from build123d import *
from OCP.BRepFilletAPI import BRepFilletAPI_MakeChamfer

# Parameters (mm, degrees)
BASE_W               = 85
BASE_H               = 100
BOSS_EXTRUDE2_DEPTH  = 2
SKETCH3_W            = 9
SKETCH3_H            = 1.5
SKETCH3_W_2          = 43
SKETCH3_H_2          = 2.5
BOSS_EXTRUDE4_DEPTH  = 11
SKETCH13_W           = 15
SKETCH13_H           = 61.230763763
SKETCH13_R           = 1
CUT_EXTRUDE2_DEPTH   = 67.537583365
SKETCH14_W           = 2.595547293
SKETCH14_H           = 6.5
SKETCH14_W_2         = 6.5
SKETCH14_H_2         = 2
BOSS_EXTRUDE5_DEPTH  = 25
SKETCH16_W           = 3.995410841
SKETCH16_H           = 2.5
BOSS_EXTRUDE6_DEPTH  = 29
SKETCH18_W           = 4
SKETCH18_H           = 6.5
BOSS_EXTRUDE7_DEPTH  = 40
CHAMFER1_SIZE        = 8.502262467
CHAMFER1_SIZE_2      = 40
SKETCH19_W           = 10.5
SKETCH19_H           = 63.5
CUT_EXTRUDE3_DEPTH   = 77.852130745
BOSS_EXTRUDE8_DEPTH  = 5
FILLET1_R            = 10
SKETCH21_W           = 2
SKETCH21_H           = 2
BOSS_EXTRUDE9_DEPTH  = 3.4
SKETCH22_W           = 64
SKETCH22_H           = 2
BOSS_EXTRUDE10_DEPTH = 35
SKETCH23_R           = 1.5
SKETCH23_W           = 30
SKETCH23_H           = 27.486629776
CUT_EXTRUDE4_DEPTH   = 104.107953137
SKETCH24_W           = 1
SKETCH24_H           = 32.46
SKETCH24_W_2         = 10
SKETCH24_H_2         = 1
BOSS_EXTRUDE11_DEPTH = 5
SKETCH26_W           = 2
SKETCH26_H           = 2
BOSS_EXTRUDE13_DEPTH = 3.4


with BuildPart() as part:
    # base → Boss-Extrude2 (new body)
    with BuildSketch(Plane(origin=(0, 0, 0), x_dir=(1, 0, 0), z_dir=(0, 1, 0))):
        Rectangle(BASE_W, BASE_H)
    extrude(amount=BOSS_EXTRUDE2_DEPTH)

    # Sketch3 → Boss-Extrude4 (add)
    with BuildSketch(Plane(origin=(0, 2, 0), x_dir=(1, 0, 0), z_dir=(0, 1, 0))):
        with Locations((38, 41.25)):
            Rectangle(SKETCH3_W, SKETCH3_H)
        with Locations((38, 27.75)):
            Rectangle(SKETCH3_W, SKETCH3_H)
        with Locations((-38, 41.25)):
            Rectangle(SKETCH3_W, SKETCH3_H)
        with Locations((-38, 27.75)):
            Rectangle(SKETCH3_W, SKETCH3_H)
        with Locations((0, 41.75)):
            Rectangle(SKETCH3_W_2, SKETCH3_H_2)
    extrude(amount=BOSS_EXTRUDE4_DEPTH)

    # Sketch13 → Cut-Extrude2 (cut, through all)
    with BuildSketch(Plane(origin=(0, 2, 0), x_dir=(1, 0, 0), z_dir=(0, 1, 0))):
        with BuildLine():
            ThreePointArc((-16.872793903, 34.5), (-13.024991104, 30.652197201), (-9.177188305, 34.5))
            Line((-9.177188305, 34.5), (-16.872793903, 34.5))
        make_face()
        with BuildLine():
            Line((-16.872793903, 34.5), (-9.177188305, 34.5))
            ThreePointArc((-9.177188305, 34.5), (-13.024991104, 38.347802799), (-16.872793903, 34.5))
        make_face()
        with BuildLine():
            ThreePointArc((9.177188305, 34.5), (13.024991104, 30.652197201), (16.872793903, 34.5))
            Line((16.872793903, 34.5), (9.177188305, 34.5))
        make_face()
        with BuildLine():
            Line((9.177188305, 34.5), (16.872793903, 34.5))
            ThreePointArc((16.872793903, 34.5), (13.024991104, 38.347802799), (9.177188305, 34.5))
        make_face()
        with Locations((-7.5, -19.384618119)):
            Rectangle(SKETCH13_W, SKETCH13_H)
        with Locations((7.5, -19.384618119)):
            Rectangle(SKETCH13_W, SKETCH13_H)
        with Locations(Location((28.5, 45, 0), (0, 0, 270))):
            Circle(SKETCH13_R)
        with Locations(Location((28.5, 24, 0), (0, 0, 90))):
            Circle(SKETCH13_R)
        with Locations(Location((-28.5, 24, 0), (0, 0, 270))):
            Circle(SKETCH13_R)
        with Locations(Location((-28.5, 45, 0), (0, 0, 90))):
            Circle(SKETCH13_R)
    extrude(amount=-CUT_EXTRUDE2_DEPTH, mode=Mode.SUBTRACT)

    # Sketch14 → Boss-Extrude5 (add)
    with BuildSketch(Plane(origin=(0, 2, 0), x_dir=(1, 0, 0), z_dir=(0, 1, 0))):
        with Locations((-36.123593927, 23.75)):
            Rectangle(SKETCH14_W, SKETCH14_H)
        with Locations((-34.171367573, 19.5)):
            Rectangle(SKETCH14_W_2, SKETCH14_H_2)
        with Locations((36.123593927, 23.75)):
            Rectangle(SKETCH14_W, SKETCH14_H)
        Polygon((37.421367573, 20.5), (34.82582028, 20.5), (30.921367573, 20.5), (30.921367573, 18.5), (37.421367573, 18.5), align=None)
    extrude(amount=BOSS_EXTRUDE5_DEPTH)

    # Sketch16 → Boss-Extrude6 (add)
    with BuildSketch(Plane(origin=(0, 13, 0), x_dir=(1, 0, 0), z_dir=(0, 1, 0))):
        with Locations((-19.50229458, 41.75)):
            Rectangle(SKETCH16_W, SKETCH16_H)
        with Locations((19.50229458, 41.75)):
            Rectangle(SKETCH16_W, SKETCH16_H)
    extrude(amount=BOSS_EXTRUDE6_DEPTH)

    # Sketch18 → Boss-Extrude7 (add)
    with BuildSketch(Plane(origin=(0, 2, 0), x_dir=(1, 0, 0), z_dir=(0, 1, 0))):
        with Locations((-19.5, 46.25)):
            Rectangle(SKETCH18_W, SKETCH18_H)
        with Locations((19.5, 46.25)):
            Rectangle(SKETCH18_W, SKETCH18_H)
    extrude(amount=BOSS_EXTRUDE7_DEPTH)

    # Chamfer1
    chamfer1_edges_1 = [part.edges().sort_by_distance(p)[0] for p in [
        (-19.5, 42, -49.5),
    ]]
    chamfer1_side_1 = [part.faces().sort_by_distance(p)[0] for p in [
        (-19.5, 42, -49.329954751),
    ]]
    chamfer1_edges_2 = [part.edges().sort_by_distance(p)[0] for p in [
        (19.5, 42, -49.5),
    ]]
    chamfer1_side_2 = [part.faces().sort_by_distance(p)[0] for p in [
        (19.5, 42, -49.329954751),
    ]]
    chamfer1 = BRepFilletAPI_MakeChamfer(part.part.solid().wrapped)
    for e in chamfer1_edges_1:
        chamfer1.Add(CHAMFER1_SIZE - 0.0001, CHAMFER1_SIZE_2 - 0.0001, e.wrapped, chamfer1_side_1[0].wrapped)
    for e in chamfer1_edges_2:
        chamfer1.Add(CHAMFER1_SIZE - 0.0001, CHAMFER1_SIZE_2 - 0.0001, e.wrapped, chamfer1_side_2[0].wrapped)
    add(Compound.cast(chamfer1.Shape()), mode=Mode.REPLACE)  # a hair under: the kernel refuses the full size

    # Sketch19 → Cut-Extrude3 (cut, through all)
    with BuildSketch(Plane(origin=(0, 2, 0), x_dir=(1, 0, 0), z_dir=(0, 1, 0))):
        with Locations((-37.25, -18.25)):
            Rectangle(SKETCH19_W, SKETCH19_H)
        with Locations((37.25, -18.25)):
            Rectangle(SKETCH19_W, SKETCH19_H)
    extrude(amount=-CUT_EXTRUDE3_DEPTH, mode=Mode.SUBTRACT)

    # Sketch20 → Boss-Extrude8 (add)
    with BuildSketch(Plane(origin=(0, 2, 0), x_dir=(1, 0, 0), z_dir=(0, 1, 0))):
        Polygon((-26, -50), (-25, -50), (-25, 18.538863673), (-20, 18.538863673), (-20, 19.538863673), (-26, 19.538863673), align=None)
        Polygon((20, 18.538863673), (25, 18.538863673), (25, -50), (26, -50), (26, 19.538863673), (20, 19.538863673), align=None)
    extrude(amount=BOSS_EXTRUDE8_DEPTH)

    # Fillet1
    fillet1_edges = [part.edges().sort_by_distance(p)[0] for p in [
        (-42.5, 1, -13.5),
        (42.5, 1, -13.5),
    ]]
    fillet(fillet1_edges, radius=FILLET1_R)

    # Sketch21 → Boss-Extrude9 (add)
    with BuildSketch(Plane(origin=(0, 2, 0), x_dir=(1, 0, 0), z_dir=(0, 1, 0))):
        with Locations((-24, 17.538863673)):
            Rectangle(SKETCH21_W, SKETCH21_H)
        with Locations((24, 17.538863673)):
            Rectangle(SKETCH21_W, SKETCH21_H)
    extrude(amount=BOSS_EXTRUDE9_DEPTH)

    # Sketch22 → Boss-Extrude10 (add)
    with BuildSketch(Plane.XY.offset(50)):
        with Locations((0, 1)):
            Rectangle(SKETCH22_W, SKETCH22_H)
    extrude(amount=BOSS_EXTRUDE10_DEPTH)

    # Sketch23 → Cut-Extrude4 (cut, through all)
    with BuildSketch(Plane(origin=(0, 2, 0), x_dir=(1, 0, 0), z_dir=(0, 1, 0))):
        with Locations(Location((18, -72, 0), (0, 0, 270))):
            Circle(SKETCH23_R)
        with Locations(Location((18, -65, 0), (0, 0, 270))):
            Circle(SKETCH23_R)
        with Locations(Location((18, -58, 0), (0, 0, 270))):
            Circle(SKETCH23_R)
        with Locations(Location((18, -51, 0), (0, 0, 270))):
            Circle(SKETCH23_R)
        with Locations(Location((-18, -51, 0), (0, 0, 90))):
            Circle(SKETCH23_R)
        with Locations(Location((-18, -58, 0), (0, 0, 90))):
            Circle(SKETCH23_R)
        with Locations(Location((-18, -65, 0), (0, 0, 90))):
            Circle(SKETCH23_R)
        with Locations(Location((-18, -72, 0), (0, 0, 90))):
            Circle(SKETCH23_R)
        with Locations((0, -61.256685112)):
            Rectangle(SKETCH23_W, SKETCH23_H)
    extrude(amount=-CUT_EXTRUDE4_DEPTH, mode=Mode.SUBTRACT)

    # Sketch24 → Boss-Extrude11 (add)
    with BuildSketch(Plane(origin=(0, 2, 0), x_dir=(1, 0, 0), z_dir=(0, 1, 0))):
        with Locations((-25.5, -66.23)):
            Rectangle(SKETCH24_W, SKETCH24_H)
        with Locations((-20, -81.96)):
            Rectangle(SKETCH24_W_2, SKETCH24_H_2)
        with Locations((25.5, -66.23)):
            Rectangle(SKETCH24_W, SKETCH24_H)
        with Locations((20, -81.96)):
            Rectangle(SKETCH24_W_2, SKETCH24_H_2)
    extrude(amount=BOSS_EXTRUDE11_DEPTH)

    # Sketch26 → Boss-Extrude13 (add)
    with BuildSketch(Plane(origin=(0, 2, 0), x_dir=(1, 0, 0), z_dir=(0, 1, 0))):
        with Locations((24, -80.46)):
            Rectangle(SKETCH26_W, SKETCH26_H)
        with Locations((-24, -80.46)):
            Rectangle(SKETCH26_W, SKETCH26_H)
    extrude(amount=BOSS_EXTRUDE13_DEPTH)


solid = part.part
Verification items for the finished model (mm, model axes). A direction names the side the tool comes from. Give positions to 0.01 mm unless a question says otherwise; leave off trailing zeros. Loops run counter-clockwise (first coordinate to the right, second up) from the corner with the lowest first, then second, coordinate; pieces in that order, holes last.
1. Go/stop test with flat-tipped pins: P1, Ø5, axis at y = 9.5, z = -23.5, coming from the -X side; P2, Ø2, axis at y = 4.5, z = 23, coming from the -X side; P3, Ø2, axis at x = -23.5, y = 4, coming from the +Z side; P4, Ø8, axis at y = 14.5, z = 39.5, coming from the -X side. Record where each tip stops, or that it passes through.
Derived:
P1: stops at x = -37.42
P2: stops at x = -26
P3: stops at z = 82.46
P4: passes through
2. Cross-section at C-C on z = 65. Record the cut outline in (x, y).
Derived:
outline: (-32, 0) - (-19.5, 0) - (-19.5, 2) - (-25, 2) - (-25, 7) - (-26, 7) - (-26, 2) - (-32, 2) - close; (-16.5, 0) - (-15, 0) - (-15, 2) - (-16.5, 2) - close; (15, 0) - (16.5, 0) - (16.5, 2) - (15, 2) - close; (19.5, 0) - (32, 0) - (32, 2) - (26, 2) - (26, 7) - (25, 7) - (25, 2) - (19.5, 2) - close
3. Material ranges on probe 1 along X at (y, z) = (1.6, -24); probe 2 along X at (y, z) = (0.6, 72); probe 3 along Z at (x, y) = (37, 4), recorded low to high.
Derived:
probe 1: x = -42.5 to -29.5, -27.5 to 27.5, 29.5 to 42.5
probe 2: x = -32 to -19.5, -16.5 to -15, 15 to 16.5, 19.5 to 32
probe 3: z = -42 to -40.5, -28.5 to -18.5
4. Cross-section at D-D on z = -34.5. Record the cut outline in (x, y).
Derived:
outline: (-42.5, 0) - (-16.87, 0) - (-16.87, 2) - (-42.5, 2) - close; (-9.18, 0) - (9.18, 0) - (9.18, 2) - (-9.18, 2) - close; (16.87, 0) - (42.5, 0) - (42.5, 2) - (16.87, 2) - close
5. Cross-section at A-A on z = 44.5. Record the cut outline in (x, y), and give its area (3 significant figures).
Derived:
outline: (-32, 0) - (-15, 0) - (-15, 2) - (-25, 2) - (-25, 7) - (-26, 7) - (-26, 2) - (-32, 2) - close; (15, 0) - (32, 0) - (32, 2) - (26, 2) - (26, 7) - (25, 7) - (25, 2) - (15, 2) - close
area: 78.0 mm2
6. Cross-section at B-B on x = -7. Record the cut outline in (y, z), and give its area (3 significant figures).
Derived:
outline: (0, -50) - (2, -50) - (2, -43) - (13, -43) - (13, -40.5) - (2, -40.5) - (2, -11.23) - (0, -11.23) - close; (0, 75) - (2, 75) - (2, 85) - (0, 85) - close
area: 125 mm2
7. Tool access check on faces 4 (the flat face through (-34.826, 14, -24)), 5 (the flat face through (-21, 4, 82.46)), 6 (the flat face through (0, 13, -42)), 7 (the flat face through (37.421, 14, -23)). Record the directions out of +Z, -Z, +X, -X, +Y, -Y that give a thin tool (end or side, any length) a straight path to the whole face; none if there is none.
Derived:
face 4: +Y
face 5: +Z, +X, -X, +Y
face 6: +Z, -Z, +Y
face 7: +Z, +X, +Y
8. Release check for a two-part mould opening along Z. For faces 1 (the flat face through (26, 4, 32)), 2 (the flat face through (-23, 4, -19.539)), 3 (the cylindrical face through (39.65, 0.99, -16.51)) record: +Z half, -Z half, draft (parallel to the pull), parting line (faces both ways), or undercut.
Derived:
face 1: draft
face 2: undercut
face 3: +Z half
